```python
from build123d import *

# Parameters (mm, degrees)
EXTRUDE_1_DEPTH = 3


with BuildPart() as part:
    # 草图1 → 凸台-拉伸1 (new body)
    with BuildSketch(Plane.XY):
        Polygon((0, 0), (-80, 0), (-145.109322536, -69.821200219), (-85, -69.821200219), (-85, -111.821200219), (0, -111.821200219), align=None)
        Polygon((80, 0), (0, 0), (0, -111.821200219), (85, -111.821200219), (85, -69.821200219), (145.109322536, -69.821200219), align=None)
    extrude(amount=EXTRUDE_1_DEPTH)


solid = part.part
```
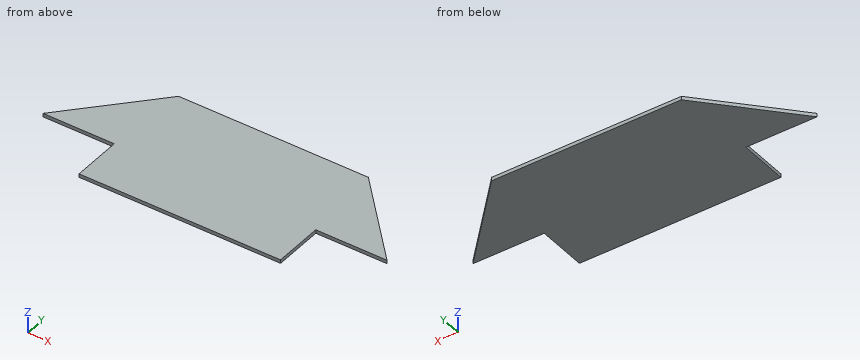
Model file for the job. Use its own axes, mm. Give positions to 0.01 mm unless a question says otherwise; leave off trailing zeros. Loops run counter-clockwise (first coordinate to the right, second up) from the corner with the lowest first, then second, coordinate; pieces in that order, holes last. Notation, with made-up numbers: M 35.5,59 L 85.5,59 A29 ccw 85.5,89 Z; hole C 66,9 d4. An arc over 180 degrees is marked long. Use one line per item in the form item = value.
Item 1: Flat gauge pins, fed straight in: pin 1 Ø0.9 at (y, z) = (-88, 1.5) entering from -X; pin 2 Ø0.9 at (x, z) = (121.5, 1) entering from -Y. Where does each tip first touch, or does it go through?
Filled in:
pin_1 = -85
pin_2 = -69.82
Item 2: Slice it at B-B on y = -95. List the corners of the cut face in (x, z).
Filled in:
outline = M -85,0 L 85,0 L 85,3 L -85,3 Z
Item 3: Slice it at A-A on z = 2.2. List the corners of the cut face in (x, y), and give its area (3 significant figures).
Filled in:
outline = M -145.11,-69.82 L -85,-69.82 L -85,-111.82 L 85,-111.82 L 85,-69.82 L 145.11,-69.82 L 80,0 L -80,0 Z
area = 22,900 mm^2
Item 4: Slice it at C-C on x = 90. List the corners of the cut face in (y, z), and give its area (3 significant figures).
Filled in:
outline = M -69.82,0 L -10.72,0 L -10.72,3 L -69.82,3 Z
area = 177 mm^2
Item 5: Drill centre lines: L1, parallel to X at y = -80.5, z = 2.15; L2, parallel to Y at x = -123.5, z = 0.85; L3, parallel to X at y = -13.5, z = 0.25. Where is each one in solid material? Low to high.
Filled in:
L1 = -85 to 85
L2 = -69.82 to -46.65
L3 = -92.59 to 92.59
